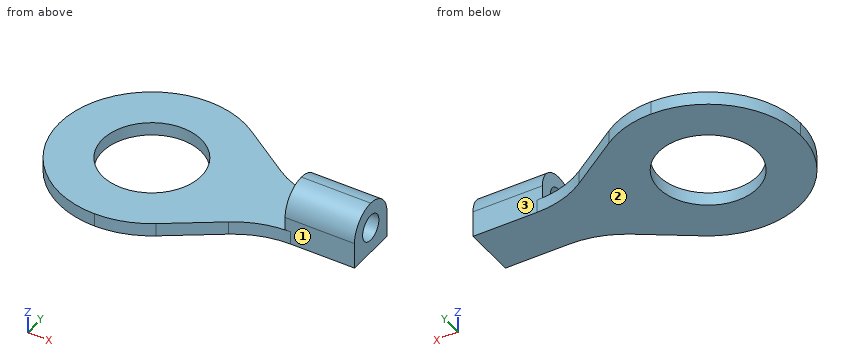
```python
from build123d import *

# Parameters (mm, degrees)
F0_R     = 3.2
F1_DEPTH = 0.85
F3_DEPTH = 2.55
F4_R     = 1.69999
F5_R     = 0.85
F6_DEPTH = 25


# Not quite as in the source:
# - a fillet or chamfer is up to 0.001 mm smaller than in the source, because OpenCascade refuses the exact size


with BuildPart() as f1:
    # F0 (on Top) → F1 (new body)
    with BuildSketch(Plane.XY):
        with BuildLine():
            Line((16.0373335058, 4.3), (20.2, 4.3))
            Line((20.2, 4.3), (20.2, 7.7))
            Line((20.2, 7.7), (16.0373335058, 7.7))
            ThreePointArc((16.0373335058, 7.7), (14.2805243712, 7.9629605488), (12.6777057346, 8.7287927785))
            Line((12.6777057346, 8.7287927785), (9.3596277711, 10.9712072215))
            ThreePointArc((9.3596277711, 10.9712072215), (7.7568091346, 11.7370394512), (6, 12))
            ThreePointArc((6, 12), (1.7573593129, 10.2426406871), (0, 6))
            ThreePointArc((0, 6), (1.7573593129, 1.7573593129), (6, 0))
            ThreePointArc((6, 0), (7.7568091346, 0.2629605488), (9.3596277711, 1.0287927785))
            Line((9.3596277711, 1.0287927785), (12.6777057346, 3.2712072215))
            ThreePointArc((12.6777057346, 3.2712072215), (14.2805243712, 4.0370394512), (16.0373335058, 4.3))
        make_face()
        with Locations((6, 6)):
            Circle(F0_R, mode=Mode.SUBTRACT)
    extrude(amount=F1_DEPTH)

    # F2 (on face) → F3 (join)
    with BuildSketch(Plane.XY.offset(0.85)):
        Polygon((20.2, 4.3), (20.2, 7.7), (16.0373335058, 7.7), (15.7, 7.7), (15.7, 4.3), (16.0373335058, 4.3), align=None)
    extrude(amount=F3_DEPTH)

    # F4 (radius 1.7 in the source; OpenCascade refuses exactly that, so slightly less here)
    f4_edges = [f1.edges().sort_by_distance(p)[0] for p in [
        (17.95, 7.7, 3.4),
        (17.95, 4.3, 3.4),
    ]]
    fillet(f4_edges, radius=F4_R)

    # F5 (on face) → F6 (cut)
    with BuildSketch(Plane.YZ.offset(20.2)):
        with Locations((6, 1.7)):
            Circle(F5_R)
    extrude(amount=-F6_DEPTH, mode=Mode.SUBTRACT)


solid = f1.part
```
Can you work these out from the model? Positions are in its coordinate system, mm. Face numbers are marked on the shaded views. A direction names the side the tool comes from. Coordinates: 2 decimals unless noted, no trailing zeros. Loops run counter-clockwise (first coordinate to the right, second up) from the corner with the lowest first, then second, coordinate; pieces in that order, holes last. Notation, with made-up numbers: M 27.5,73.25 L 68.5,73.25 A8 ccw 68.5,82.25 Z; hole C -0.75,36 d1. An arc over 180 degrees is marked long. Put each result on its own line as item: value. Start each with the question number.
(1) Imagine slicing it at B-B on x = 7. List the corners of the cut face in (y, z) for me.
(2) Imagine slicing it at C-C on z = 1.9. List the corners of the cut face in (x, y) for me.
(3) Which directions (+Z, -Z, +X, -X, +Y, -Y) give clear straight access to the entire face, cutting with the end or side of a thin tool? Please do the marked faces 1, 2 and 3.
(4) Imagine slicing it at D-D on y = 9.75. List the corners of the cut face in (x, z) for me.
(5) Imagine slicing it at A-A on z = 0.6. List the corners of the cut face in (x, y) for me, and give its area (3 significant figures).
(6) I need wall thicknesses on probe 1 along Y at (x, z) = (18.7, 1.7); probe 2 along Y at (x, z) = (6, 0.5); probe 3 along Z at (x, y) = (2.5, 2). Which ranges of each line are inside material? Lowest first, please.
(7) Will these pins go through, and if not, where does the flat tip stop? pin 1 Ø1.4 at (x, z) = (18, 1) entering from +Y; pin 2 Ø1.9 at (x, z) = (17.5, 0.5) entering from -Y.
Worked answers:
1. outline: M 0.08,0 L 2.96,0 L 2.96,0.85 L 0.08,0.85 Z; M 9.04,0 L 11.92,0 L 11.92,0.85 L 9.04,0.85 Z
2. outline: M 15.7,4.31 L 20.2,4.31 L 20.2,5.17 L 15.7,5.17 Z; M 15.7,6.83 L 20.2,6.83 L 20.2,7.69 L 15.7,7.69 Z
3. face 1: +Z, -Z, +X, -Y
3. face 2: -Z, +X, -X, +Y, -Y
3. face 3: +Z, -Z, +X, +Y
4. outline: M 1.32,0 L 11.17,0 L 11.17,0.85 L 1.32,0.85 Z
5. outline: M 9.36,1.03 L 12.68,3.27 A6 cw 16.04,4.3 L 20.2,4.3 L 20.2,7.7 L 16.04,7.7 A6 cw 12.68,8.73 L 9.36,10.97 A6 ccw long Z; hole C 6,6 d6.4
5. area: 116 mm2
6. probe 1: y = 4.3 to 5.15, 6.85 to 7.7
6. probe 2: y = 0 to 2.8, 9.2 to 12
6. probe 3: z = 0 to 0.85
7. pin 1: stops at y = 7.7
7. pin 2: stops at y = 4.3
